from build123d import *

# Parameters (mm, degrees)
EXTRUDE_1_DEPTH     = 80
FILLET_1_R          = 1
CUT_EXTRUDE_1_DEPTH = 10


with BuildPart() as part:
    # 草图1 → 凸台-拉伸1 (new body)
    with BuildSketch(Plane(origin=(0, 0, 0), x_dir=(0, 0, -1), z_dir=(1, 0, 0))):
        Polygon((0, -10), (0, 10), (6.5, 13.120839269), (6.5, 17.5), (5.5, 17.5), (5.5, 13.75), (-1, 10.629160731), (-1, -10.629160731), (5.5, -13.75), (5.5, -17.5), (6.5, -17.5), (6.5, -13.120839269), align=None)
    extrude(amount=EXTRUDE_1_DEPTH)

    # 圆角1
    fillet_1_edges = [part.edges().sort_by_distance(p)[0] for p in [
        (40, 10, 0),
        (40, -13.120839269, -6.5),
        (40, -13.75, -5.5),
        (40, -10.629160731, 1),
        (40, 10.629160731, 1),
        (40, 13.75, -5.5),
        (40, 13.120839269, -6.5),
    ]]
    fillet(fillet_1_edges, radius=FILLET_1_R)

    # 草图2 → 切除-拉伸1 (cut)
    with BuildSketch(Plane(origin=(0, 0, 0), x_dir=(-1, 0, 0), z_dir=(0, 0, -1))):
        with BuildLine():
            Line((-10, -2), (-17.5, -2))
            ThreePointArc((-17.5, -2), (-19.5, 0), (-17.5, 2))
            Line((-17.5, 2), (-10, 2))
            ThreePointArc((-10, 2), (-8, 0), (-10, -2))
        make_face()
        with BuildLine():
            Line((-30, -2), (-37.5, -2))
            ThreePointArc((-37.5, -2), (-39.5, 0), (-37.5, 2))
            Line((-37.5, 2), (-30, 2))
            ThreePointArc((-30, 2), (-28, 0), (-30, -2))
        make_face()
        with BuildLine():
            Line((-54, -2), (-61.5, -2))
            ThreePointArc((-61.5, -2), (-63.5, 0), (-61.5, 2))
            Line((-61.5, 2), (-54, 2))
            ThreePointArc((-54, 2), (-52, 0), (-54, -2))
        make_face()
        with BuildLine():
            Line((-74, -2), (-81.5, -2))
            ThreePointArc((-81.5, -2), (-83.5, 0), (-81.5, 2))
            Line((-81.5, 2), (-74, 2))
            ThreePointArc((-74, 2), (-72, 0), (-74, -2))
        make_face()
        with BuildLine():
            Line((-98, -2), (-105.5, -2))
            ThreePointArc((-105.5, -2), (-107.5, 0), (-105.5, 2))
            Line((-105.5, 2), (-98, 2))
            ThreePointArc((-98, 2), (-96, 0), (-98, -2))
        make_face()
        with BuildLine():
            Line((-118, -2), (-125.5, -2))
            ThreePointArc((-125.5, -2), (-127.5, 0), (-125.5, 2))
            Line((-125.5, 2), (-118, 2))
            ThreePointArc((-118, 2), (-116, 0), (-118, -2))
        make_face()
        with BuildLine():
            Line((-142, -2), (-149.5, -2))
            ThreePointArc((-149.5, -2), (-151.5, 0), (-149.5, 2))
            Line((-149.5, 2), (-142, 2))
            ThreePointArc((-142, 2), (-140, 0), (-142, -2))
        make_face()
        with BuildLine():
            Line((-162, -2), (-169.5, -2))
            ThreePointArc((-169.5, -2), (-171.5, 0), (-169.5, 2))
            Line((-169.5, 2), (-162, 2))
            ThreePointArc((-162, 2), (-160, 0), (-162, -2))
        make_face()
        with BuildLine():
            Line((-186, -2), (-193.5, -2))
            ThreePointArc((-193.5, -2), (-195.5, 0), (-193.5, 2))
            Line((-193.5, 2), (-186, 2))
            ThreePointArc((-186, 2), (-184, 0), (-186, -2))
        make_face()
        with BuildLine():
            Line((-206, -2), (-213.5, -2))
            ThreePointArc((-213.5, -2), (-215.5, 0), (-213.5, 2))
            Line((-213.5, 2), (-206, 2))
            ThreePointArc((-206, 2), (-204, 0), (-206, -2))
        make_face()
        with BuildLine():
            Line((-230, -2), (-237.5, -2))
            ThreePointArc((-237.5, -2), (-239.5, 0), (-237.5, 2))
            Line((-237.5, 2), (-230, 2))
            ThreePointArc((-230, 2), (-228, 0), (-230, -2))
        make_face()
        with BuildLine():
            Line((-250, -2), (-257.5, -2))
            ThreePointArc((-257.5, -2), (-259.5, 0), (-257.5, 2))
            Line((-257.5, 2), (-250, 2))
            ThreePointArc((-250, 2), (-248, 0), (-250, -2))
        make_face()
        with BuildLine():
            Line((-274, -2), (-281.5, -2))
            ThreePointArc((-281.5, -2), (-283.5, 0), (-281.5, 2))
            Line((-281.5, 2), (-274, 2))
            ThreePointArc((-274, 2), (-272, 0), (-274, -2))
        make_face()
        with BuildLine():
            Line((-294, -2), (-301.5, -2))
            ThreePointArc((-301.5, -2), (-303.5, 0), (-301.5, 2))
            Line((-301.5, 2), (-294, 2))
            ThreePointArc((-294, 2), (-292, 0), (-294, -2))
        make_face()
        with BuildLine():
            Line((-318, -2), (-325.5, -2))
            ThreePointArc((-325.5, -2), (-327.5, 0), (-325.5, 2))
            Line((-325.5, 2), (-318, 2))
            ThreePointArc((-318, 2), (-316, 0), (-318, -2))
        make_face()
        with BuildLine():
            Line((-338, -2), (-345.5, -2))
            ThreePointArc((-345.5, -2), (-347.5, 0), (-345.5, 2))
            Line((-345.5, 2), (-338, 2))
            ThreePointArc((-338, 2), (-336, 0), (-338, -2))
        make_face()
        with BuildLine():
            Line((-362, -2), (-369.5, -2))
            ThreePointArc((-369.5, -2), (-371.5, 0), (-369.5, 2))
            Line((-369.5, 2), (-362, 2))
            ThreePointArc((-362, 2), (-360, 0), (-362, -2))
        make_face()
        with BuildLine():
            Line((-382, -2), (-389.5, -2))
            ThreePointArc((-389.5, -2), (-391.5, 0), (-389.5, 2))
            Line((-389.5, 2), (-382, 2))
            ThreePointArc((-382, 2), (-380, 0), (-382, -2))
        make_face()
    extrude(amount=-CUT_EXTRUDE_1_DEPTH, mode=Mode.SUBTRACT)


solid = part.part
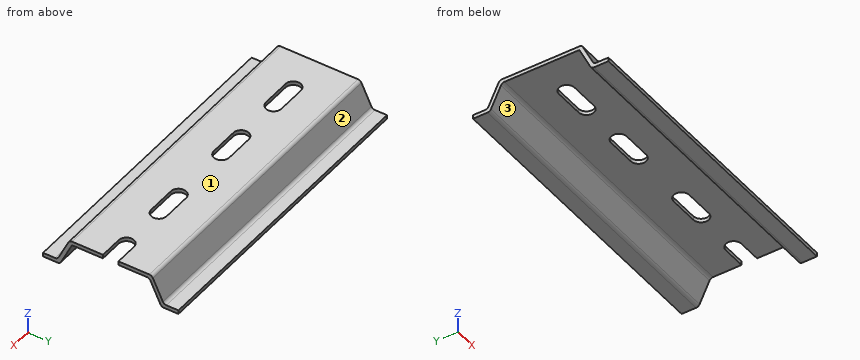
Design review of the part built by this model. Coordinates are the model's own, in mm. Face numbers are marked on the shaded views. Round coordinates to 2 decimals unless told otherwise and drop trailing zeros. Write each loop counter-clockwise with the first axis right and the second up, starting at its lowest first coordinate (ties: lowest second). Pieces come first, ordered by that corner, then holes.
Item 1: Wall thickness on L1, parallel to Y at x = 59, z = -4.75; L2, parallel to Z at x = 25, y = 0.5; L3, parallel to Y at x = 54, z = -2.5: over which ranges is each line inside the solid? List them lowest first.
Item 2: Draft analysis for pull direction Y (two halves, no side actions). For the marked faces 1, 2 and 3, state which applies: released by +Y, released by -Y, zero draft, split by the parting line, or undercut.
Item 3: For pin 1 Ø0.5 at (x, z) = (34, 0.5) entering from +Y; pin 2 Ø15.5 at (x, y) = (33.5, 3) entering from -Z; pin 3 Ø0.5 at (x, z) = (58.5, 0.5) entering from -Y, all flat-tipped, find the tip position at first contact; note any pin that passes through.
Item 4: Consider section B-B on z = -3.25. Give the boundary of the cut face in (x, y).
Item 5: Consider section D-D on x = 49. Give the boundary of the cut face in (y, z).
Item 6: Consider section C-C on x = 62.5. Give the boundary of the cut face in (y, z).
Item 7: Consider section A-A on y = 0. Give the boundary of the cut face in (x, z).
Check values:
1. L1: y = -13.39 to -12.28, 12.28 to 13.39
1. L2: z = 0 to 1
1. L3: y = -12.31 to -11.2, 11.2 to 12.31
2. face 1: zero draft
2. face 2: released by +Y
2. face 3: undercut
3. pin 1: stops at y = 10.99
3. pin 2: stops at z = -1.56
3. pin 3: stops at y = -10.99
4. outline: (0, -12.67) - (80, -12.67) - (80, -11.56) - (0, -11.56) - close; (0, 11.56) - (80, 11.56) - (80, 12.67) - (0, 12.67) - close
5. outline: (-17.5, -6.5) - (-13.75, -6.5) arc R1 ccw to (-12.85, -5.93) - (-10, 0) - (9.37, 0) arc R1 cw to (10.27, -0.57) - (12.85, -5.93) arc R1 ccw to (13.75, -6.5) - (17.5, -6.5) - (17.5, -5.5) - (14.38, -5.5) arc R1 cw to (13.48, -4.93) - (10.9, 0.43) arc R1 ccw to (10, 1) - (-10, 1) arc R1 ccw to (-10.9, 0.43) - (-13.48, -4.93) arc R1 cw to (-14.38, -5.5) - (-17.5, -5.5) - close
6. outline: (-17.5, -6.5) - (-13.75, -6.5) arc R1 ccw to (-12.85, -5.93) - (-10, 0) - (-1.73, 0) - (-1.73, 1) - (-10, 1) arc R1 ccw to (-10.9, 0.43) - (-13.48, -4.93) arc R1 cw to (-14.38, -5.5) - (-17.5, -5.5) - close; (1.73, 0) - (9.37, 0) arc R1 cw to (10.27, -0.57) - (12.85, -5.93) arc R1 ccw to (13.75, -6.5) - (17.5, -6.5) - (17.5, -5.5) - (14.38, -5.5) arc R1 cw to (13.48, -4.93) - (10.9, 0.43) arc R1 ccw to (10, 1) - (1.73, 1) - close
7. outline: (0, 0) - (8, 0) - (8, 1) - (0, 1) - close; (19.5, 0) - (28, 0) - (28, 1) - (19.5, 1) - close; (39.5, 0) - (52, 0) - (52, 1) - (39.5, 1) - close; (63.5, 0) - (72, 0) - (72, 1) - (63.5, 1) - close
